from build123d import *

# Parameters (mm, degrees)
F3_DEPTH  = 36.957
F4_R      = 6.35
F7_DEPTH  = 5.1562
F8_R      = 5.15619
F11_DEPTH = 5.1562
F12_R     = 5.15619


# Not quite as in the source:
# - a fillet or chamfer is up to 0.001 mm smaller than in the source, because OpenCascade refuses the exact size


with BuildPart() as f1:
    # F0 (on Front) → F1 (revolve)
    with BuildSketch(Plane.XZ):
        Polygon((-88.2352406061, 116.84), (-77.6180406061, 106.2228), (-63.2924406061, 106.2228), (-52.6752406061, 116.84), (-43.7044062913, 116.84), (-43.7044062913, 106.5403), (70.0067593939, 106.5403), (70.0067593939, 106.2228), (161.4467593939, 106.2228), (161.4467593939, 114.4397), (70.0067593939, 114.4397), (70.0067593939, 120.523), (-108.0472406061, 120.523), (-108.0472406061, 116.84), align=None)
    revolve(axis=Axis((26.6997593939, 0, 0), (1, 0, 0)))

    # F2 (on Right) → F3 (cut, symmetric)
    with BuildSketch(Plane.YZ):
        with BuildLine():
            Line((-79.5165483207, 101.776540644), (-60.0681501855, 76.8837261913))
            ThreePointArc((-60.0681501855, 76.8837261913), (24.428788043, 94.4591146185), (89.8107580216, 38.1224050048))
            Line((89.8107580216, 38.1224050048), (118.8889862246, 50.465380577))
            ThreePointArc((118.8889862246, 50.465380577), (32.3381508976, 125.0423515407), (-79.5165483207, 101.776540644))
        make_face()
        with BuildLine():
            ThreePointArc((60.0681501855, -76.8837261913), (-24.428788043, -94.4591146185), (-89.8107580216, -38.1224050048))
            Line((-89.8107580216, -38.1224050048), (-118.8889862246, -50.465380577))
            ThreePointArc((-118.8889862246, -50.465380577), (-32.3381508976, -125.0423515407), (79.5165483207, -101.776540644))
            Line((79.5165483207, -101.776540644), (60.0681501855, -76.8837261913))
        make_face()
    extrude(amount=F3_DEPTH, both=True, mode=Mode.SUBTRACT)

    # F4
    f4_edges = [f1.edges().sort_by_distance(p)[0] for p in [
        (36.957, -69.897063, 89.464161),
        (-36.957, -69.897063, 89.464161),
        (-36.957, 104.506435, 44.36035),
        (36.957, 104.506435, 44.36035),
        (36.957, -104.506435, -44.36035),
        (36.957, 69.897063, -89.464161),
        (-36.957, -104.506435, -44.36035),
        (-36.957, 69.897063, -89.464161),
    ]]
    fillet(f4_edges, radius=F4_R)

    # F6 (on offset) → F7 (cut, symmetric)
    with BuildSketch(Plane.YZ.offset(9.017)):
        with BuildLine():
            ThreePointArc((93.8788780653, -25.1547695639), (84.169499428, -48.5952831523), (68.7241085014, -68.7241085014))
            Line((68.7241085014, -68.7241085014), (90.3596269568, -90.3596269568))
            ThreePointArc((90.3596269568, -90.3596269568), (110.6674896962, -63.8939049666), (123.4335458995, -33.0739189427))
            Line((123.4335458995, -33.0739189427), (93.8788780653, -25.1547695639))
        make_face()
        with BuildLine():
            ThreePointArc((-92.7935106347, 24.8639462374), (-83.1963856114, 48.0334556284), (-67.9295643973, 67.9295643973))
            Line((-67.9295643973, 67.9295643973), (-89.4286909818, 89.4286909818))
            ThreePointArc((-89.4286909818, 89.4286909818), (-109.5273306353, 63.2356338259), (-122.1618637084, 32.7331727265))
            Line((-122.1618637084, 32.7331727265), (-92.7935106347, 24.8639462374))
        make_face()
    extrude(amount=F7_DEPTH, both=True, mode=Mode.SUBTRACT)

    # F8 (radius 5.1562 in the source; OpenCascade refuses exactly that, so slightly less here)
    f8_edges = [f1.edges().sort_by_distance(p)[0] for p in [
        (14.1732, 80.279, -80.279),
        (3.8608, 80.279, -80.279),
        (3.8608, -80.279, 80.279),
        (14.1732, -80.279, 80.279),
    ]]
    fillet(f8_edges, radius=F8_R)

    # F10 (on offset) → F11 (cut, symmetric)
    with BuildSketch(Plane.YZ.offset(57.277)):
        with BuildLine():
            ThreePointArc((64.781849813, 77.2040022495), (80.3789780557, 60.7977459719), (91.9209264172, 41.3241976951))
            Line((91.9209264172, 41.3241976951), (115.0678452351, 52.1177832026))
            ThreePointArc((115.0678452351, 52.1177832026), (100.6398977696, 76.3445041239), (81.1972614412, 96.7671280314))
            Line((81.1972614412, 96.7671280314), (64.781849813, 77.2040022495))
        make_face()
        with BuildLine():
            ThreePointArc((-62.1507050275, -74.0683259988), (-76.7088050422, -58.8607363245), (-87.6302951199, -40.8626777008))
            Line((-87.6302951199, -40.8626777008), (-116.6783232789, -54.4079956856))
            ThreePointArc((-116.6783232789, -54.4079956856), (-102.1365355533, -78.3721201887), (-82.7526604046, -98.6207803339))
            Line((-82.7526604046, -98.6207803339), (-62.1507050275, -74.0683259988))
        make_face()
    extrude(amount=F11_DEPTH, both=True, mode=Mode.SUBTRACT)

    # F12 (radius 5.1562 in the source; OpenCascade refuses exactly that, so slightly less here)
    f12_edges = [f1.edges().sort_by_distance(p)[0] for p in [
        (62.4332, 72.976738, 86.97029),
        (52.1208, 72.976738, 86.97029),
        (62.4332, -72.976738, -86.97029),
        (52.1208, -72.976738, -86.97029),
    ]]
    fillet(f12_edges, radius=F12_R)


solid = f1.part
The model under review builds one solid part; all positions refer to its coordinate system, in mm. A direction names the side the tool comes from. Give positions to 0.01 mm unless a question says otherwise; leave off trailing zeros. Write each loop counter-clockwise with the first axis right and the second up, starting at its lowest first coordinate (ties: lowest second). Pieces come first, ordered by that corner, then holes.
1. Add section A-A, the plane x = -15. Write out the cut boundary in (y, z).
2. Add section C-C, the plane y = 0. Count the separate pieces of the cut face and the enclosed holes in it, plus the area to 3 significant figures.
3. Wall thickness on L1, parallel to Y at x = -95, z = -2; L2, parallel to Z at x = -94, y = 0; L3, parallel to Z at x = -66, y = 0: over which ranges is each line inside the solid? List them lowest first.
4. Tool access review of faces 1 (the flat face through (8.94, 109.76, -29.41)), 2 (the cylindrical face through (-35.05, 68.35, -90.43)), 3 (the conical face through (-62.63, -32.11, 101.95)): name each direction out of +Z, -Z, +X, -X, +Y, -Y from which nothing blocks a thin tool from reaching the whole face with its end or side.
5. Add section B-B, the plane z = 0. Write out the cut boundary in (x, y), plus the area to 3 significant figures.
6. Draft analysis for pull direction Y (two halves, no side actions). For faces 4 (the flat face through (-0.428, 104.416, 44.322)), 5 (the cylindrical face through (12.623, -81.344, 79.265)), 6 (the cylindrical face through (60.96, 74.06, 85.85)), state which applies: +Y half, -Y half, draft (parallel to the pull), parting line (faces both ways), or undercut.
7. Add section D-D, the plane x = 111. Write out the cut boundary in (y, z).
8. For P1, Ø11, axis at y = 91, z = 58.5, coming from the -X side; P2, Ø3, axis at x = 21.5, z = 12, coming from the +Y side; P3, Ø10, axis at x = 42, z = -28, coming from the -Y side; P4, Ø12, axis at x = 28.5, y = 32, coming from the +Z side, all flat-tipped, find the tip position at first contact; note any pin that passes through.
Worked answers:
1. outline: (-110.94, -47.09) - (-98.07, -41.63) arc R106.54 cw to (-65.59, 83.95) - (-74.2, 94.97) arc R120.52 ccw to start; (65.59, -83.95) - (74.2, -94.97) arc R120.52 ccw to (110.94, 47.09) - (98.07, 41.63) arc R106.54 cw to start
2. separate pieces: 4
2. enclosed holes: 0
2. area: 3,620 mm2
3. L1: y = -120.51 to -116.82, 116.82 to 120.51
3. L2: z = -120.52 to -116.84, 116.84 to 120.52
3. L3: z = -120.52 to -106.22, 106.22 to 120.52
4. face 1: -Z
4. face 2: -Z, -Y
4. face 3: none
5. outline: (-108.05, -120.52) - (70.01, -120.52) - (70.01, -114.44) - (161.45, -114.44) - (161.45, -106.22) - (70.01, -106.22) - (70.01, -106.54) - (-43.7, -106.54) - (-43.7, -116.84) - (-52.68, -116.84) - (-63.29, -106.22) - (-77.62, -106.22) - (-88.24, -116.84) - (-108.05, -116.84) - close; (-108.05, 116.84) - (-88.24, 116.84) - (-77.62, 106.22) - (-63.29, 106.22) - (-52.68, 116.84) - (-43.7, 116.84) - (-43.7, 106.54) - (70.01, 106.54) - (70.01, 106.22) - (161.45, 106.22) - (161.45, 114.44) - (70.01, 114.44) - (70.01, 120.52) - (-108.05, 120.52) - close
5. area: 5,690 mm2
6. face 4: undercut
6. face 5: -Y half
6. face 6: +Y half
7. outline: circle Ø228.88 at (0, 0); hole circle Ø212.45 at (0, 0)
8. P1: stops at x = -85.08
8. P2: stops at y = 120.06
8. P3: stops at y = -118.31
8. P4: passes through
